from build123d import *

# Parameters (mm, degrees)
F1_DEPTH = 10
F3_DEPTH = 14
F5_DEPTH = 12


with BuildPart() as f1:
    # F0 (on Front) → F1 (new body, symmetric)
    with BuildSketch(Plane.XZ):
        with BuildLine():
            ThreePointArc((12.7872340426, -15.3781223022), (0, -20), (-12.7872340426, -15.3781223022))
            ThreePointArc((-12.7872340426, -15.3781223022), (-17.7161714029, -15.8315277476), (-17.2627659574, -20.760465108))
            ThreePointArc((-17.2627659574, -20.760465108), (0, -27), (17.2627659574, -20.760465108))
            ThreePointArc((17.2627659574, -20.760465108), (17.7161714029, -15.8315277476), (12.7872340426, -15.3781223022))
        make_face()
        with BuildLine():
            ThreePointArc((-13.525, -18.0692937051), (-13.6063617319, -18.556597988), (-13.8416206189, -18.9910383771))
            ThreePointArc((-13.8416206189, -18.9910383771), (-16.4436382681, -17.5819894221), (-13.525, -18.0692937051))
        make_face(mode=Mode.SUBTRACT)
        with BuildLine():
            ThreePointArc((16.525, -18.0692937051), (15.512304283, -19.4879319732), (13.8416206189, -18.9910383771))
            ThreePointArc((13.8416206189, -18.9910383771), (14.537695717, -16.6506554369), (16.525, -18.0692937051))
        make_face(mode=Mode.SUBTRACT)
    extrude(amount=F1_DEPTH, both=True)

    # F2 (on face) → F3 (cut)
    with BuildSketch(Plane.XZ.offset(10)):
        Polygon((-2.3909412976, -9.4292996609), (-9.1462977059, -30.4901171085), (24.7288569808, -31.99012205), (30.0422031432, -11.7994137108), align=None)
    extrude(amount=-F3_DEPTH, mode=Mode.SUBTRACT)

    # F4 (on face) → F5 (cut)
    with BuildSketch(Plane(origin=(0, 10, 0), x_dir=(-1, 0, 0), z_dir=(0, 1, 0))):
        Polygon((13.4975397959, -6.4067570493), (6.4347200096, -13.4695768356), (17.8041364998, -28.4565351903), (37.6144833863, -8.6461873725), align=None)
    extrude(amount=-F5_DEPTH, mode=Mode.SUBTRACT)


solid = f1.part
Input: part model. Units: mm. Frame: model coordinates. A direction names the side the tool comes from. Round coordinates to 2 decimals unless told otherwise and drop trailing zeros. Order: outer loops, then holes, each group sorted by start corner. A loop starts at its lowest first (then second) coordinate and runs counter-clockwise, first axis right, second up.
1. Mould query, pull axis Z, two halves, no side actions, for faces 1 (the face through (-14.219, -5.944, -19.334)), 2 (the face through (-11.652, 4.084, -20.346)), 3 (the face through (2, 10, -22)). Classes: released by +Z, released by -Z, zero draft, split by the parting line, or undercut.
The answers:
face 1: undercut
face 2: released by +Z
face 3: zero draft
2. Cut plane D-D, the plane z = -21.5. Output: boundary loops of the cut face in (x, y), then the cut area to 3 significant figures.
The answers:
outline: (-16.33, -10) - (-6.26, -10) - (-6.26, 4) - (16.33, 4) - (16.33, 10) - (-12.53, 10) - (-12.53, -2) - (-16.33, -2) - close
area: 291 mm2
3. Cut plane A-A, the plane z = -15.75. Output: boundary loops of the cut face in (x, y).
The answers:
outline: (-17.65, -10) - (-12.33, -10) - (-12.33, -2) - (-17.65, -2) - close; (12.33, 4) - (17.65, 4) - (17.65, 10) - (12.33, 10) - close
4. Material intervals for line 1 (Y direction, x = -14, z = -16.5); line 2 (X direction, y = 7, z = -18); line 3 (Z direction, x = -15.5, y = -2.25), sorted ascending.
The answers:
line 1: y = -10 to -2
line 2: x = -9.87 to -8.72, 8.72 to 13.53, 16.52 to 18.52
line 3: z = -22.11 to -19.49, -16.65 to -14.6
5. Pin query (flat end, axial travel): P1, Ø1.5, axis at y = -0.5, z = -25.5, coming from the -X side; P2, Ø1.8, axis at x = -15.03, z = -18.07, coming from the -Y side; P3, Ø1.5, axis at y = 2.5, z = -21.5, coming from the +X side; P4, Ø1, axis at x = -4, z = -25.5, coming from the -Y side. Return the tip coordinate at first contact, or that it passes through.
The answers:
P1: stops at x = -10.79
P2: passes through
P3: stops at x = -6.02
P4: stops at y = 4
6. Cut plane B-B, the plane y = -6. Output: boundary loops of the cut face in (x, z) (3 decimals), then the cut area to 3 significant figures.
The answers:
outline: (-17.263, -20.76) arc R27 ccw to (-7.67, -25.888) - (-5.531, -19.22) arc R20 cw to (-12.787, -15.378) arc R3.5 ccw to start; hole circle Ø3 at (-15.025, -18.069)
area: 79.4 mm2
7. Cut plane C-C, the plane x = -14.5. Output: boundary loops of the cut face in (y, z), then the cut area to 3 significant figures.
The answers:
outline: (-10, -22.78) - (-2, -22.78) - (-2, -19.47) - (-10, -19.47) - close; (-10, -16.66) - (-2, -16.66) - (-2, -14.61) - (-10, -14.61) - close
area: 42.9 mm2
8. Set-up query: faces 4 (the face through (-14, -2, -20)), 5 (the face through (-17.666, -6.056, -15.773)), 6 (the face through (-6.586, -3.098, -22.507)). Return all of +Z, -Z, +X, -X, +Y, -Y with unobstructed straight access to the full face (end or side cutting, diameter ignored); none if empty.
The answers:
face 4: +Z, -X, +Y
face 5: +Y, -Y
face 6: -Z, +X, -Y
